```python
from build123d import *

# Parameters (mm, degrees)
SKETCH1_W           = 81
SKETCH1_H           = 41
BOSS_EXTRUDE1_DEPTH = 2
SKETCH2_R           = 3
CUT_EXTRUDE1_DEPTH  = 0.5
SKETCH3_R           = 1.5
CUT_EXTRUDE2_DEPTH  = 91.797852398
SKETCH4_R           = 3
BOSS_EXTRUDE2_DEPTH = 2


with BuildPart() as part:
    # Sketch1 → Boss-Extrude1 (new body)
    with BuildSketch(Plane(origin=(0, 0, 0), x_dir=(1, 0, 0), z_dir=(0, 1, 0))):
        with Locations((40.5, 20.5)):
            Rectangle(SKETCH1_W, SKETCH1_H)
    extrude(amount=BOSS_EXTRUDE1_DEPTH)

    # Sketch2 → Cut-Extrude1 (cut)
    with BuildSketch(Plane(origin=(0, 2, 0), x_dir=(1, 0, 0), z_dir=(0, 1, 0))):
        with Locations(Location((20.5, 20.5, 0), (0, 0, 270))):
            Circle(SKETCH2_R)
        with Locations(Location((60.5, 20.5, 0), (0, 0, 270))):
            Circle(SKETCH2_R)
    extrude(amount=-CUT_EXTRUDE1_DEPTH, mode=Mode.SUBTRACT)

    # Sketch3 → Cut-Extrude2 (cut, through all)
    with BuildSketch(Plane(origin=(0, 1.5, 0), x_dir=(1, 0, 0), z_dir=(0, 1, 0))):
        with Locations(Location((20.5, 20.5, 0), (0, 0, 270))):
            Circle(SKETCH3_R)
        with Locations(Location((60.5, 20.5, 0), (0, 0, 270))):
            Circle(SKETCH3_R)
    extrude(amount=-CUT_EXTRUDE2_DEPTH, mode=Mode.SUBTRACT)

    # Sketch4 → Boss-Extrude2 (add)
    with BuildSketch(Plane.XZ):
        with Locations(Location((70.5, -30.5, 0), (0, 0, 270))):
            Circle(SKETCH4_R)
        with Locations(Location((50.5, -30.5, 0), (0, 0, 270))):
            Circle(SKETCH4_R)
        with Locations(Location((30.5, -30.5, 0), (0, 0, 270))):
            Circle(SKETCH4_R)
        with Locations(Location((10.5, -30.5, 0), (0, 0, 270))):
            Circle(SKETCH4_R)
        with Locations(Location((50.5, -10.5, 0), (0, 0, 270))):
            Circle(SKETCH4_R)
        with Locations(Location((30.5, -10.5, 0), (0, 0, 270))):
            Circle(SKETCH4_R)
        with Locations(Location((10.5, -10.5, 0), (0, 0, 270))):
            Circle(SKETCH4_R)
        with Locations(Location((70.5, -10.5, 0), (0, 0, 270))):
            Circle(SKETCH4_R)
    extrude(amount=BOSS_EXTRUDE2_DEPTH)


solid = part.part
```
Check sheet for the modelled part. Datum: model origin and axes. Units: mm. A direction names the side the tool comes from. Give positions to 0.01 mm unless a question says otherwise; leave off trailing zeros. Write each loop counter-clockwise with the first axis right and the second up, starting at its lowest first coordinate (ties: lowest second). Pieces come first, ordered by that corner, then holes. Notation, with made-up numbers: (25, 8) - (70, 8) arc R28 ccw to (70, 32) - close; hole circle Ø6 at (57, 51). An arc over 180 degrees is marked (long way). Answer as a JSON object with one key per item and string values. Group by question number.
1) Sectioned sample at B-B (x = 60.5). Record the cut outline in (y, z), then the cut area to 3 significant figures.
2) Depth check by flat-ended pin: P1, Ø5.5, axis at x = 20.5, z = -20.5, coming from the +Y side; P2, Ø5, axis at x = 60.5, z = -20.5, coming from the -Y side; P3, Ø9.5, axis at x = 60.5, z = -20.5, coming from the +Y side. Enter the tip coordinate at first touch or a pass-through.
3) Release check for a two-part mould opening along X. For faces 1 (the face through (59, 1.5, -19)), 2 (the face through (71, -2, -10)), 3 (the face through (81, 1, -20)) record: pulls with the +X half, pulls with the -X half, needs draft (parallel to the pull), parting line crosses it, or undercut.
4) Sectioned sample at C-C (z = -10.5). Record the cut outline in (x, y).
5) Access from +Z, -Z, +X, -X, +Y, -Y to the whole of each face (thin tool, end or side, straight path). Record for faces 4 (the face through (62.53, 1.75, -22.71)), 5 (the face through (30.6, -1, -27.5)), 6 (the face through (51, -2, -10)).
6) Sectioned sample at D-D (x = 50.5). Record the cut outline in (y, z), then the cut area to 3 significant figures.
7) Sectioned sample at A-A (y = -1.3). Record the cut outline in (x, z), then the cut area to 3 significant figures.
8) Thickness scan on probe 1 along X at (y, z) = (1, -20.5); probe 2 along Y at (x, z) = (64.5, -14); probe 3 along Y at (x, z) = (60, -18). Record the ranges inside material, lowest first. Write a range as from..to.
Geometry results:
{
 "1": {"outline": "(0, -41) - (2, -41) - (2, -23.5) - (1.5, -23.5) - (1.5, -22) - (0, -22) - close; (0, -19) - (1.5, -19) - (1.5, -17.5) - (2, -17.5) - (2, 0) - (0, 0) - close", "area": "74.5 mm^2"},
 "2": {"P1": "stops at y = 1.5", "P2": "stops at y = 0", "P3": "stops at y = 2"},
 "3": {"face 1": "undercut", "face 2": "needs draft", "face 3": "pulls with the +X half"},
 "4": {"outline": "(0, 0) - (7.5, 0) - (7.5, -2) - (13.5, -2) - (13.5, 0) - (27.5, 0) - (27.5, -2) - (33.5, -2) - (33.5, 0) - (47.5, 0) - (47.5, -2) - (53.5, -2) - (53.5, 0) - (67.5, 0) - (67.5, -2) - (73.5, -2) - (73.5, 0) - (81, 0) - (81, 2) - (0, 2) - close"},
 "5": {"face 4": "+Y", "face 5": "-Y", "face 6": "+Z, -Z, +X, -X, -Y"},
 "6": {"outline": "(-2, -33.5) - (0, -33.5) - (0, -41) - (2, -41) - (2, 0) - (0, 0) - (0, -7.5) - (-2, -7.5) - (-2, -13.5) - (0, -13.5) - (0, -27.5) - (-2, -27.5) - close", "area": "106 mm^2"},
 "7": {"outline": "circle Ø6 at (10.5, -30.5); circle Ø6 at (10.5, -10.5); circle Ø6 at (30.5, -30.5); circle Ø6 at (30.5, -10.5); circle Ø6 at (50.5, -30.5); circle Ø6 at (50.5, -10.5); circle Ø6 at (70.5, -30.5); circle Ø6 at (70.5, -10.5)", "area": "226 mm^2"},
 "8": {"probe 1": "x = 0..19, 22..59, 62..81", "probe 2": "y = 0..2", "probe 3": "y = 0..1.5"}
}
